from build123d import *

# Parameters (mm, degrees)
F0_W     = 37.55
F0_H     = 26.23
F0_W_2   = 27.55
F0_H_2   = 16.23
F1_DEPTH = 13
F2_W     = 61.55
F2_H     = 13
F2_R     = 2.1
F3_DEPTH = 5
F4_R     = 3
F5_R     = 1.5
F6_R     = 5
F7_R     = 5


with BuildPart() as f1:
    # F0 (on Front) → F1 (new body)
    with BuildSketch(Plane.XZ):
        Rectangle(F0_W, F0_H)
        Rectangle(F0_W_2, F0_H_2, mode=Mode.SUBTRACT)
    extrude(amount=F1_DEPTH)

    # F2 (on face) → F3 (join)
    with BuildSketch(Plane.XY.offset(13.115)):
        with Locations((0, -6.5)):
            Rectangle(F2_W, F2_H)
        with Locations((-24.775, -6.5)):
            Circle(F2_R, mode=Mode.SUBTRACT)
        with Locations((24.775, -6.5)):
            Circle(F2_R, mode=Mode.SUBTRACT)
    extrude(amount=-F3_DEPTH)

    # F4
    f4_edges = [f1.edges().sort_by_distance(p)[0] for p in [
        (-18.775, -6.5, 8.115),
        (18.775, -6.5, 8.115),
    ]]
    fillet(f4_edges, radius=F4_R)

    # F5
    f5_edges = [f1.edges().sort_by_distance(p)[0] for p in [
        (-13.775, -6.5, 8.115),
        (13.775, -6.5, 8.115),
        (13.775, -6.5, -8.115),
        (-13.775, -6.5, -8.115),
    ]]
    fillet(f5_edges, radius=F5_R)

    # F6
    f6_edges = [f1.edges().sort_by_distance(p)[0] for p in [
        (18.775, -6.5, -13.115),
        (-18.775, -6.5, -13.115),
    ]]
    fillet(f6_edges, radius=F6_R)

    # F7
    f7_edges = [f1.edges().sort_by_distance(p)[0] for p in [
        (30.775, -13, 10.615),
        (30.775, 0, 10.615),
        (-30.775, -13, 10.615),
        (-30.775, 0, 10.615),
    ]]
    fillet(f7_edges, radius=F7_R)


solid = f1.part
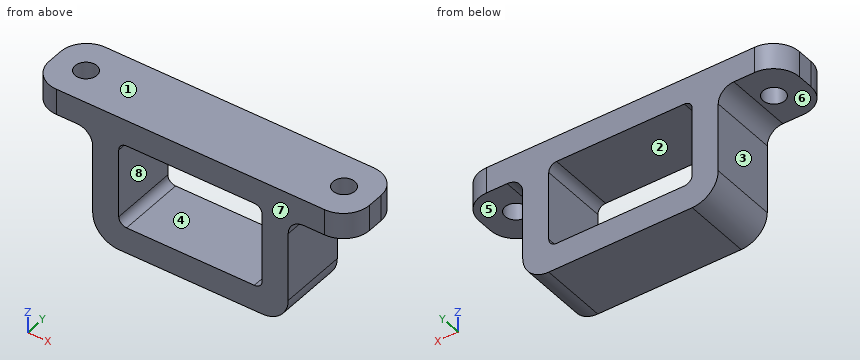
Part model, mm, in its own coordinate system. Face numbers are marked on the shaded views. A direction names the side the tool comes from. Coordinates: 2 decimals unless noted, no trailing zeros. Order: outer loops, then holes, each group sorted by start corner. A loop starts at its lowest first (then second) coordinate and runs counter-clockwise, first axis right, second up. Notation, with made-up numbers: (-39.5, 70) - (18.5, 70) arc R30 cw to (18.5, 93) - close; hole circle Ø9 at (-29, 61.25). An arc over 180 degrees is marked (long way). Use CSV: the item, a comma, the result in double quotes.
Item 1: Drop flat-ended pins along their axis: P1, Ø2, axis at y = -2, z = -4.5, coming from the -X side (3 decimals); P2, Ø8, axis at x = 1, z = -2, coming from the -Y side (3 decimals); P3, Ø3, axis at y = -5.5, z = -2.5, coming from the +X side (3 decimals); P4, Ø4.5, axis at x = 26, y = -5.5, coming from the -Z side (3 decimals). Give the stop position or say it passes through.
Solved:
P1,"stops at x = -18.775"
P2,"passes through"
P3,"stops at x = 18.775"
P4,"stops at z = 8.115"
Item 2: 3-axis set-ups, long thin cutter, end or side, ignore diameter. For the marked faces 5, 6, 7 and 8: which of +Z, -Z, +X, -X, +Y, -Y reach the whole face in a straight line?
Solved:
face 5,"-Z, +X, +Y, -Y"
face 6,"-Z, -X, +Y, -Y"
face 7,"+Z, -Z, +X, -X, -Y"
face 8,"+Y, -Y"
Item 3: Saw through at D-D on y = -10.25. Give the cut face in (x, z) (3 decimals).
Solved:
outline,"(-30.24, 8.115) - (-21.775, 8.115) arc R3 cw to (-18.775, 5.115) - (-18.775, -8.115) arc R5 ccw to (-13.775, -13.115) - (13.775, -13.115) arc R5 ccw to (18.775, -8.115) - (18.775, 5.115) arc R3 cw to (21.775, 8.115) - (30.24, 8.115) - (30.24, 13.115) - (-30.24, 13.115) - close; hole (-13.775, -6.615) arc R1.5 ccw to (-12.275, -8.115) - (12.275, -8.115) arc R1.5 ccw to (13.775, -6.615) - (13.775, 6.615) arc R1.5 ccw to (12.275, 8.115) - (-12.275, 8.115) arc R1.5 ccw to (-13.775, 6.615) - close"
Item 4: Saw through at B-B on x = 1.5. Give the cut face in (y, z) (3 decimals), and give its area (3 significant figures).
Solved:
outline,"(-13, -13.115) - (0, -13.115) - (0, -8.115) - (-13, -8.115) - close; (-13, 8.115) - (0, 8.115) - (0, 13.115) - (-13, 13.115) - close"
area,"130 mm²"
Item 5: Saw through at C-C on z = -1.5. Give the cut face in (x, y) (3 decimals).
Solved:
outline,"(-18.775, -13) - (-13.775, -13) - (-13.775, 0) - (-18.775, 0) - close; (13.775, -13) - (18.775, -13) - (18.775, 0) - (13.775, 0) - close"
Item 6: Mould opens along Z. For the marked faces 1, 2, 3 and 4 say: +Z half, -Z half, draft (parallel to the pull), parting line (faces both ways), or undercut.
Solved:
face 1,"+Z half"
face 2,"undercut"
face 3,"draft"
face 4,"undercut"
Item 7: Probe probe 1 along Z at (x, y) = (3, -4) (3 decimals); probe 2 along X at (y, z) = (-1.5, -1.5) (3 decimals); probe 3 along Z at (x, y) = (-14, -3.5) (3 decimals). List the from-to ranges inside material, lowest first.
Solved:
probe 1,"z = -13.115 to -8.115, 8.115 to 13.115"
probe 2,"x = -18.775 to -13.775, 13.775 to 18.775"
probe 3,"z = -13.11 to 13.115"
Item 8: Saw through at A-A on y = -6.5. Give the cut face in (x, z) (3 decimals), and give its area (3 significant figures).
Solved:
outline,"(-30.775, 8.115) - (-26.875, 8.115) - (-26.875, 13.115) - (-30.775, 13.115) - close; (-22.675, 8.115) - (-21.775, 8.115) arc R3 cw to (-18.775, 5.115) - (-18.775, -8.115) arc R5 ccw to (-13.775, -13.115) - (13.775, -13.115) arc R5 ccw to (18.775, -8.115) - (18.775, 5.115) arc R3 cw to (21.775, 8.115) - (22.675, 8.115) - (22.675, 13.115) - (-22.675, 13.115) - close; (26.875, 8.115) - (30.775, 8.115) - (30.775, 13.115) - (26.875, 13.115) - close; hole (-13.775, -6.615) arc R1.5 ccw to (-12.275, -8.115) - (12.275, -8.115) arc R1.5 ccw to (13.775, -6.615) - (13.775, 6.615) arc R1.5 ccw to (12.275, 8.115) - (-12.275, 8.115) arc R1.5 ccw to (-13.775, 6.615) - close"
area,"611 mm²"
